The model under review builds one solid part; all positions refer to its coordinate system, in mm. Face numbers are marked on the shaded views. A direction names the side the tool comes from. Round coordinates to 2 decimals unless told otherwise and drop trailing zeros. Order: outer loops, then holes, each group sorted by start corner. A loop starts at its lowest first (then second) coordinate and runs counter-clockwise, first axis right, second up.
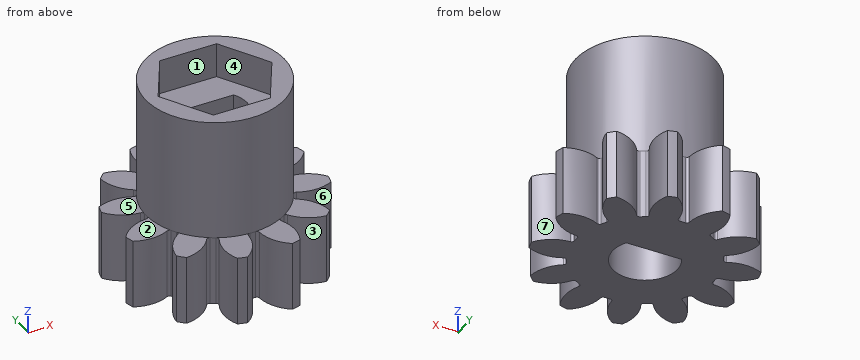
```python
from build123d import *

# Parameters (mm, degrees)
SKETCH1_R           = 6
SKETCH1_R_2         = 2
BOSS_EXTRUDE1_DEPTH = 4
CUT_EXTRUDE2_DEPTH  = 5
CIRPATTERN2_COUNT   = 12
SKETCH11_R          = 4
BOSS_EXTRUDE2_DEPTH = 11
CUT_EXTRUDE3_START  = 11
CUT_EXTRUDE3_DEPTH  = 2
CUT_EXTRUDE4_DEPTH  = 12


with BuildPart() as part:
    # Sketch1 → Boss-Extrude1 (new body)
    with BuildSketch(Plane.XY):
        Circle(SKETCH1_R)
        Circle(SKETCH1_R_2, mode=Mode.SUBTRACT)
    extrude(amount=BOSS_EXTRUDE1_DEPTH)

    # Sketch4 → Cut-Extrude2 (cut, through all)
    with BuildSketch(Plane.XY):
        with BuildLine():
            ThreePointArc((-0.160215471, 3.996790087), (-0.266788325, 4.035374045), (-0.315943185, 4.137502858))
            ThreePointArc((-0.315943185, 4.137502858), (-0.829511973, 5.435929685), (-2.010193861, 6.181352655))
            ThreePointArc((-2.010193861, 6.181352655), (0, 6.5), (2.010193861, 6.181352655))
            ThreePointArc((2.010193861, 6.181352655), (0.829511973, 5.435929685), (0.315943185, 4.137502858))
            ThreePointArc((0.315943185, 4.137502858), (0.266788325, 4.035374045), (0.160215471, 3.996790087))
            ThreePointArc((0.160215471, 3.996790087), (0, 4), (-0.160215471, 3.996790087))
        make_face()
    cut_extrude2 = extrude(amount=CUT_EXTRUDE2_DEPTH, mode=Mode.SUBTRACT)

    # CirPattern2: Cut-Extrude2 ×12 about axis
    cirpattern2_axis = Axis((0, 0, 0), (0, 0, 1))
    for i in range(1, CIRPATTERN2_COUNT):
        add(cut_extrude2.rotate(cirpattern2_axis, i * 360 / CIRPATTERN2_COUNT), mode=Mode.SUBTRACT)

    # Sketch11 → Boss-Extrude2 (add)
    with BuildSketch(Plane.XY):
        Circle(SKETCH11_R)
    extrude(amount=BOSS_EXTRUDE2_DEPTH)

    # Sketch12 → Cut-Extrude3 (cut)
    with BuildSketch(Plane.XY.offset(CUT_EXTRUDE3_START)):
        Polygon((3.290896534, 0), (1.645448267, 2.85), (-1.645448267, 2.85), (-3.290896534, 0), (-1.645448267, -2.85), (1.645448267, -2.85), align=None)
    extrude(amount=-CUT_EXTRUDE3_DEPTH, mode=Mode.SUBTRACT)

    # Sketch13 → Cut-Extrude4 (cut, through all)
    with BuildSketch(Plane.XY):
        with BuildLine():
            Line((1.6, 0.95), (-1.6, 0.95))
            ThreePointArc((-1.6, 0.95), (0, -1.860779407), (1.6, 0.95))
        make_face()
    extrude(amount=CUT_EXTRUDE4_DEPTH, mode=Mode.SUBTRACT)


solid = part.part
```
(1) Consider section A-A (x = 0). Write out the cut boundary in (y, z), and give its area (3 significant figures).
Data:
outline: (-4, 0) - (-1.86, 0) - (-1.86, 9) - (-2.85, 9) - (-2.85, 11) - (-4, 11) - close; (0.95, 0) - (4, 0) - (4, 11) - (2.85, 11) - (2.85, 9) - (0.95, 9) - close
area: 51.3 mm2
(2) Insertion check: pin 1 (0.6 mm diameter, centred on x = -1.5, y = -5, fed in from +Z); pin 2 (1.6 mm diameter, centred on x = 0.5, z = 10, fed in from +Y); pin 3 (1 mm diameter, centred on y = -3, z = 9.5, fed in from +X). Each pin has a flat end and moves straight along its axis. Give the tip position at first contact, or say it passes through.
Data:
pin 1: stops at z = 4
pin 2: stops at y = 4
pin 3: stops at x = 3.12
(3) Consider section C-C (y = 0.75). Write out the cut boundary in (x, z), and give its area (3 significant figures).
Data:
outline: (-5.33, 0) - (-1.7, 0) - (-1.7, 9) - (-2.86, 9) - (-2.86, 11) - (-3.93, 11) - (-3.93, 4) - (-5.33, 4) - close; (1.7, 0) - (5.33, 0) - (5.33, 4) - (3.93, 4) - (3.93, 11) - (2.86, 11) - (2.86, 9) - (1.7, 9) - close
area: 55.6 mm2
(4) Consider section D-D (x = 2.75). Write out the cut boundary in (y, z).
Data:
outline: (-3.89, 0) - (3.89, 0) - (3.89, 4) - (2.9, 4) - (2.9, 11) - (0.94, 11) - (0.94, 9) - (-0.94, 9) - (-0.94, 11) - (-2.9, 11) - (-2.9, 4) - (-3.89, 4) - close
(5) To check wall thickness, follow probe 1 along Y at (x, z) = (0, 3); probe 2 along X at (y, z) = (0, 6.5); probe 3 along Y at (x, z) = (3.75, 3). State the ranges of each line that lie inside material, in increasing order.
Data:
probe 1: y = -4 to -1.86, 0.95 to 4
probe 2: x = -4 to -1.86, 1.86 to 4
probe 3: y = -4.38 to -2.6, -1.8 to 1.8, 2.6 to 4.38
(6) Draft analysis for pull direction Y (two halves, no side actions). For the marked faces 1, 2 and 3, state which applies: pulls with the +Y half, pulls with the -Y half, needs draft (parallel to the pull), parting line crosses it, or undercut.
Data:
face 1: undercut
face 2: needs draft
face 3: pulls with the -Y half
(7) Consider section B-B (z = 9.5). Write out the cut boundary in (x, y).
Data:
outline: circle Ø8 at (0, 0); hole (-3.29, 0) - (-1.65, -2.85) - (1.65, -2.85) - (3.29, 0) - (1.65, 2.85) - (-1.65, 2.85) - close
(8) For the marked faces 4, 5, 6 and 7, list the 3-axis set-ups (+Z, -Z, +X, -X, +Y, -Y) from which the entire face can be reached by the end or side of a thin tool; tool diameter is ignored.
Data:
face 4: +Z
face 5: +Z, -X, +Y
face 6: +Z, -Z
face 7: +Z, -Z, +X
